from build123d import *

# Parameters (mm, degrees)
F1_W      = 660
F1_H      = 500
F1_W_2    = 560
F1_H_2    = 400
F2_DEPTH  = 25
F4_W      = 660
F4_H      = 500
F4_W_2    = 560
F4_H_2    = 400
F5_DEPTH  = 25
F8_W      = 660
F8_H      = 550
F8_W_2    = 610
F8_H_2    = 500
F9_DEPTH  = 50
F10_W     = 660
F10_H     = 550
F10_W_2   = 610
F10_H_2   = 500
F11_DEPTH = 50


with BuildPart() as f2:
    # F1 (on offset) → F2 (new body)
    with BuildSketch(Plane.XY.offset(275)):
        Rectangle(F1_W, F1_H)
        Rectangle(F1_W_2, F1_H_2, mode=Mode.SUBTRACT)
    extrude(amount=-F2_DEPTH)



with BuildPart() as f5:
    # F4 (on offset) → F5 (new body)
    with BuildSketch(Plane.XY.offset(-275)):
        Rectangle(F4_W, F4_H)
        Rectangle(F4_W_2, F4_H_2, mode=Mode.SUBTRACT)
    extrude(amount=F5_DEPTH)


with BuildPart() as f2_1:
    add(f2.part)

    add(f5.part)  # F9 merges F5
    # F8 (on offset) → F9 (join)
    with BuildSketch(Plane.XZ.offset(250)):
        Rectangle(F8_W, F8_H)
        Rectangle(F8_W_2, F8_H_2, mode=Mode.SUBTRACT)
    extrude(amount=-F9_DEPTH)

    # F10 (on offset) → F11 (join)
    with BuildSketch(Plane.XZ.offset(-250)):
        Rectangle(F10_W, F10_H)
        Rectangle(F10_W_2, F10_H_2, mode=Mode.SUBTRACT)
    extrude(amount=F11_DEPTH)


solid = f2_1.part
Model file for the job. Use its own axes, mm. A direction names the side the tool comes from. Round coordinates to 2 decimals unless told otherwise and drop trailing zeros. Order: outer loops, then holes, each group sorted by start corner. A loop starts at its lowest first (then second) coordinate and runs counter-clockwise, first axis right, second up.
(1) Drill centre line: line 1 (Z direction, x = -107, y = -211). Where is it in solid material? Low to high.
(2) Band-saw the part on C-C (y = 212.5). List the corners of the cut face in (x, z).
(3) Band-saw the part on B-B (x = -142.5). List the corners of the cut face in (y, z), then the cut area to 3 significant figures.
(4) Pull direction Z, two halves, no side cores. Call faces 5 (the face through (-26, -250, 264)), 6 (the face through (-305, -225, -3)): released by +Z, released by -Z, zero draft, split by the parting line, or undercut.
(5) Band-saw the part on A-A (y = 13.5). List the corners of the cut face in (x, z).
(6) 3-axis set-ups, long thin cutter, end or side, ignore diameter. For faces 1 (the face through (317, -200, 4)), 2 (the face through (-4, -200, -263)), 3 (the face through (305, -225, -3)), 4 (the face through (-26, 250, 264)): which of +Z, -Z, +X, -X, +Y, -Y reach the whole face in a straight line?
Verdict:
1. line 1: z = -275 to -250, 250 to 275
2. outline: (-330, -275) - (330, -275) - (330, 275) - (-330, 275) - close; hole (-305, -250) - (305, -250) - (305, 250) - (-305, 250) - close
3. outline: (-250, -275) - (-200, -275) - (-200, -250) - (-250, -250) - close; (-250, 250) - (-200, 250) - (-200, 275) - (-250, 275) - close; (200, -275) - (250, -275) - (250, -250) - (200, -250) - close; (200, 250) - (250, 250) - (250, 275) - (200, 275) - close
3. area: 5,000 mm2
4. face 5: zero draft
4. face 6: undercut
5. outline: (-330, -275) - (-280, -275) - (-280, -250) - (-330, -250) - close; (-330, 250) - (-280, 250) - (-280, 275) - (-330, 275) - close; (280, -275) - (330, -275) - (330, -250) - (280, -250) - close; (280, 250) - (330, 250) - (330, 275) - (280, 275) - close
6. face 1: +X, -X
6. face 2: +Z, -Z
6. face 3: +Y, -Y
6. face 4: +Z, -Z, +X, -X, +Y
